from build123d import *

# Parameters (mm, degrees)
EXTRUIR_L_MINA1_DEPTH = 20


with BuildPart() as part:
    # Croquis2 → Extruir-Lámina1 (new body)
    with BuildSketch(Plane.XY):
        with BuildLine():
            Line((-429.684186478, -78.209898266), (-374.32854171, -126.474819196))
            ThreePointArc((-374.32854171, -126.474819196), (-356.25601454, -133.247210514), (-338.183487369, -126.474819196))
            Line((-338.183487369, -126.474819196), (-282.827842602, -78.209898266))
            ThreePointArc((-282.827842602, -78.209898266), (-279.664968242, -76.346198087), (-276.042663992, -75.749486696))
            Line((-276.042663992, -75.749486696), (-42.376100513, -80.735910629))
            ThreePointArc((-42.376100513, -80.735910629), (11.241002289, -28.807937643), (-41.256010137, 24.252139416))
            Line((-41.256010137, 24.252139416), (-671.256009706, 24.252139416))
            ThreePointArc((-671.256009706, 24.252139416), (-723.753022133, -28.807937666), (-670.135919286, -80.735910628))
            Line((-670.135919286, -80.735910628), (-436.469365096, -75.749486696))
            ThreePointArc((-436.469365096, -75.749486696), (-432.847060841, -76.346198085), (-429.684186478, -78.209898266))
        make_face()
        with BuildLine():
            Line((-426.398272447, -74.441242142), (-371.042627679, -122.706163072))
            ThreePointArc((-371.042627679, -122.706163072), (-356.25601454, -128.247210514), (-341.4694014, -122.706163072))
            Line((-341.4694014, -122.706163072), (-286.113756633, -74.441242142))
            ThreePointArc((-286.113756633, -74.441242142), (-281.369445094, -71.645691873), (-275.935988718, -70.750624787))
            Line((-275.935988718, -70.750624787), (-42.269425239, -75.73704872))
            ThreePointArc((-42.269425239, -75.73704872), (6.24128682, -28.754596971), (-41.256010137, 19.252139416))
            Line((-41.256010137, 19.252139416), (-671.256009706, 19.252139416))
            ThreePointArc((-671.256009706, 19.252139416), (-718.753306663, -28.754596991), (-670.242594564, -75.737048719))
            Line((-670.242594564, -75.737048719), (-436.576040374, -70.750624787))
            ThreePointArc((-436.576040374, -70.750624787), (-431.142583991, -71.645691871), (-426.398272447, -74.441242142))
        make_face(mode=Mode.SUBTRACT)
    extrude(amount=-EXTRUIR_L_MINA1_DEPTH)


solid = part.part
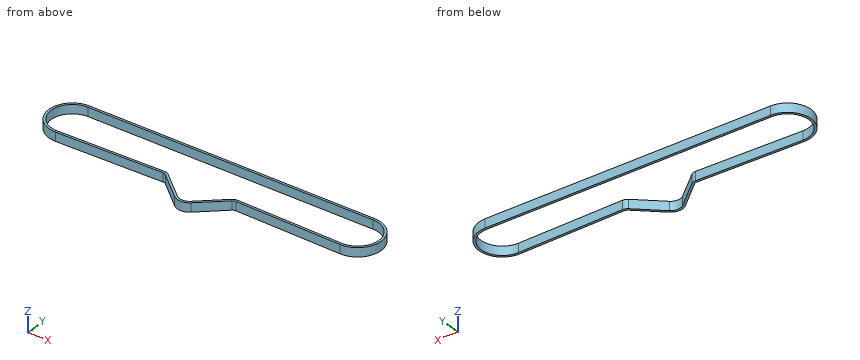
Here's how the part is built. I have some questions about the finished solid (model axes, mm). Coordinates: 2 decimals unless noted, no trailing zeros. Loops run counter-clockwise (first coordinate to the right, second up) from the corner with the lowest first, then second, coordinate; pieces in that order, holes last.
1. Imagine slicing it at A-A, the plane y = -25.5. Please give me the cut outline in (x, z).
2. For P1, Ø6, axis at y = 0.5, z = -4.5, coming from the +X side; P2, Ø5, axis at y = -108.5, z = -14.5, coming from the +X side; P3, Ø10, axis at y = -105.5, z = -11, coming from the -X side, each with a flat end and sliding along its axis, tell me the tip position at first contact or that it passes through.
3. I need wall thicknesses on L1, parallel to X at y = -123, z = -3.25; L2, parallel to X at y = -60.5, z = -11; L3, parallel to Y at x = -368.5, z = -5.25. Which ranges of each line are inside material? Lowest first, please.
4. Imagine slicing it at B-B, the plane x = -109. Please give me the cut outline in (y, z), and give its area (3 significant figures).
5. Imagine slicing it at C-C, the plane z = -15.5. Please give me the cut outline in (x, y).
Taken from the geometry:
1. outline: (-723.68, -20) - (-718.68, -20) - (-718.68, 0) - (-723.68, 0) - close; (6.16, -20) - (11.17, -20) - (11.17, 0) - (6.16, 0) - close
2. P1: stops at x = 4.5
2. P2: stops at x = -314.7
2. P3: stops at x = -404.12
3. L1: x = -378.31 to -370.7, -341.81 to -334.2
3. L2: x = -712.68 to -706.13, -6.38 to 0.17
3. L3: y = -130.37 to -124.62, 19.25 to 24.25
4. outline: (-79.31, -20) - (-74.31, -20) - (-74.31, 0) - (-79.31, 0) - close; (19.25, -20) - (24.25, -20) - (24.25, 0) - (19.25, 0) - close
4. area: 200 mm2
5. outline: (-671.26, 24.25) arc R52.5 ccw (long way) to (-670.14, -80.74) - (-436.47, -75.75) arc R10 cw to (-429.68, -78.21) - (-374.33, -126.47) arc R27.5 ccw to (-338.18, -126.47) - (-282.83, -78.21) arc R10 cw to (-276.04, -75.75) - (-42.38, -80.74) arc R52.5 ccw (long way) to (-41.26, 24.25) - close; hole (-671.26, 19.25) arc R47.5 ccw (long way) to (-670.24, -75.74) - (-436.58, -70.75) arc R15 cw to (-426.4, -74.44) - (-371.04, -122.71) arc R22.5 ccw to (-341.47, -122.71) - (-286.11, -74.44) arc R15 cw to (-275.94, -70.75) - (-42.27, -75.74) arc R47.5 ccw (long way) to (-41.26, 19.25) - close
